CAD build for the part. Positions are in the model's coordinates, mm. A direction names the side the tool comes from. Round coordinates to 2 decimals unless told otherwise and drop trailing zeros. Loops run counter-clockwise (first coordinate to the right, second up) from the corner with the lowest first, then second, coordinate; pieces in that order, holes last. Notation, with made-up numbers: M -35.5,88.5 L -29.5,88.5 A26 cw -29.5,119.5 Z; hole C -28.5,32.5 d3. An arc over 180 degrees is marked long. One line per item, written item: value. Start each with the question number.
from build123d import *

# Parameters (mm, degrees)
EXTRUDE_1_DEPTH          = 8
CUT_EXTRUDE_1_DEPTH      = 24.556069282
CUT_EXTRUDE_2_REACH      = 25.556
SKETCH_3_W               = 11.85
SKETCH_3_H               = 2.762520892
SKETCH_3_H_2             = 2.75
CUT_EXTRUDE_3_DEPTH      = 10
CUT_EXTRUDE_3_DEPTH_BACK = 3
SKETCH_4_W               = 1.2
SKETCH_4_H               = 1.4
SKETCH_4_W_2             = 0.9
SKETCH_4_H_2             = 1.28
SKETCH_4_H_3             = 0.95
SKETCH_5_R               = 0.35
EXTRUDE_2_DEPTH          = 4.8
CUT_EXTRUDE_4_DEPTH      = 1
SKETCH_7_W               = 4.4
SKETCH_7_H               = 5.2
CUT_EXTRUDE_5_DEPTH      = 19.930728988
SKETCH_8_W               = 1.6
SKETCH_8_H               = 1.6
SKETCH_8_W_2             = 1.55
SKETCH_8_H_2             = 5.8
CUT_EXTRUDE_6_DEPTH      = 1.5


with BuildPart() as part:
    # 草图1 → 凸台-拉伸1 (new, symmetric)
    with BuildSketch(Plane.XY):
        Polygon((-0.75, 5.1), (0.8, 5.1), (0.8, 2.6), (0, 2.6), (0, -2.6), (3, -2.6), (3, -6.1), (0.15, -6.1), (0.15, -8.2), (-0.75, -8.2), (-0.75, -3.25), (-9.45, -3.25), (-9.45, -8.2), (-10.65, -8.2), (-10.65, -6.1), (-17.72, -6.1), (-17.72, -2.6), (-10.25, -2.6), (-10.25, 2.6), (-11.05, 2.6), (-11.05, 5.1), (-9.45, 5.1), (-9.45, 3.25), (-0.75, 3.25), align=None)
    extrude(amount=EXTRUDE_1_DEPTH, both=True)

    # 草图2 → 切除-拉伸1 (cut, through all)
    with BuildSketch(Plane(origin=(0, 5.1, 0), x_dir=(1, 0, 0), z_dir=(0, 1, 0))):
        Polygon((-11.05, 8.719427198), (-0.75, 8.719427198), (-0.75, 2.8), (-9.45, 2.8), (-9.45, 5.25), (-11.05, 5.25), align=None)
        Polygon((-11.05, -8), (-0.75, -8), (-0.75, -2.8), (-9.45, -2.8), (-9.45, -5.25), (-11.05, -5.25), align=None)
    extrude(amount=-CUT_EXTRUDE_1_DEPTH, mode=Mode.SUBTRACT)

    # 切除-拉伸2: up to this face of the body (flat: up to its plane)
    cut_extrude_2_end = Plane(part.part.faces().sort_by_distance((-14.112466991, -2.6, 0))[0])
    # 草图3 → 切除-拉伸2 (cut, up to the picked face)
    with BuildSketch(Plane(origin=(0, 5.1, 0), x_dir=(1, 0, 0), z_dir=(0, 1, 0)), mode=Mode.PRIVATE) as cut_extrude_2_sk1:
        with Locations((-5.125, 6.618739554)):
            Rectangle(SKETCH_3_W, SKETCH_3_H)
    cut_extrude_2_tool1 = split(extrude(cut_extrude_2_sk1.sketch, amount=-CUT_EXTRUDE_2_REACH, mode=Mode.PRIVATE), bisect_by=cut_extrude_2_end, keep=Keep.BOTH, mode=Mode.PRIVATE)
    # 草图3 → 切除-拉伸2 (cut, up to the picked face)
    with BuildSketch(Plane(origin=(0, 5.1, 0), x_dir=(1, 0, 0), z_dir=(0, 1, 0)), mode=Mode.PRIVATE) as cut_extrude_2_sk2:
        with Locations((-5.125, -6.625)):
            Rectangle(SKETCH_3_W, SKETCH_3_H_2)
    cut_extrude_2_tool2 = split(extrude(cut_extrude_2_sk2.sketch, amount=-CUT_EXTRUDE_2_REACH, mode=Mode.PRIVATE), bisect_by=cut_extrude_2_end, keep=Keep.BOTH, mode=Mode.PRIVATE)
    add(cut_extrude_2_tool1.solids().sort_by(Axis((-5.125, 5.1, -6.61874), (0, -1, 0)))[0], mode=Mode.SUBTRACT)
    add(cut_extrude_2_tool2.solids().sort_by(Axis((-5.125, 5.1, 6.625), (0, -1, 0)))[0], mode=Mode.SUBTRACT)

    # 草图4 → 切除-拉伸3 (cut, two sides: drawn at the far end of the back side and taken through both)
    with BuildSketch(Plane.XZ.offset(6.1).offset(-CUT_EXTRUDE_3_DEPTH_BACK)):
        with Locations((-10.05, 1.6)):
            Rectangle(SKETCH_4_W, SKETCH_4_H)
        with Locations((-10.05, -1.6)):
            Rectangle(SKETCH_4_W, SKETCH_4_H)
        with Locations((-0.3, 2.88)):
            Rectangle(SKETCH_4_W_2, SKETCH_4_H_2)
        with Locations((-0.3, -2.88)):
            Rectangle(SKETCH_4_W_2, SKETCH_4_H_2)
        with Locations((-0.3, 0)):
            Rectangle(SKETCH_4_W_2, SKETCH_4_H_2)
        with Locations((-0.3, 5.76)):
            Rectangle(SKETCH_4_W_2, SKETCH_4_H_2)
        with Locations((-0.3, -5.76)):
            Rectangle(SKETCH_4_W_2, SKETCH_4_H_2)
        with Locations((-10.05, 4.775)):
            Rectangle(SKETCH_4_W, SKETCH_4_H_3)
        with Locations((-10.05, -4.775)):
            Rectangle(SKETCH_4_W, SKETCH_4_H_3)
    extrude(amount=CUT_EXTRUDE_3_DEPTH + CUT_EXTRUDE_3_DEPTH_BACK, mode=Mode.SUBTRACT)

    # 草图5 → 凸台-拉伸2 (add)
    with BuildSketch(Plane.XZ.offset(6.1)):
        with Locations(Location((-15.65, 0, 0), (0, 0, 90))):
            Circle(SKETCH_5_R)
        with Locations(Location((-15.65, 3.2, 0), (0, 0, 90))):
            Circle(SKETCH_5_R)
        with Locations(Location((-15.65, 6.4, 0), (0, 0, 90))):
            Circle(SKETCH_5_R)
        with Locations(Location((-15.65, -3.2, 0), (0, 0, 90))):
            Circle(SKETCH_5_R)
        with Locations(Location((-15.65, -6.4, 0), (0, 0, 90))):
            Circle(SKETCH_5_R)
        with Locations(Location((1.75, 6.4, 0), (0, 0, 180))):
            Circle(SKETCH_5_R)
        with Locations(Location((1.75, 3.2, 0), (0, 0, 180))):
            Circle(SKETCH_5_R)
        with Locations(Location((1.75, 0, 0), (0, 0, 180))):
            Circle(SKETCH_5_R)
        with Locations(Location((1.75, -3.2, 0), (0, 0, 180))):
            Circle(SKETCH_5_R)
        with Locations(Location((1.75, -6.4, 0), (0, 0, 180))):
            Circle(SKETCH_5_R)
    extrude(amount=EXTRUDE_2_DEPTH)

    # 草图6 → 切除-拉伸4 (cut)
    with BuildSketch(Plane.XZ.offset(6.1)):
        Polygon((-16.22, 2.137501461), (-13.276335298, 2.137501461), (-15.965272543, 5.540797618), (-14.866770258, 6.408721998), (-11.492087758, 2.137501461), (-10.65, 2.137501461), (-10.65, 0.737501461), (-16.22, 0.737501461), align=None)
        Polygon((-16.22, -0.737501461), (-10.65, -0.737501461), (-10.65, -2.503069938), (-11.492087758, -2.503069938), (-14.964878351, -6.426327028), (-15.965272543, -5.540797618), (-13.276335298, -2.503069938), (-16.22, -2.503069938), align=None)
    extrude(amount=-CUT_EXTRUDE_4_DEPTH, mode=Mode.SUBTRACT)

    # 草图7 → 切除-拉伸5 (cut, through all)
    with BuildSketch(Plane.ZY.offset(10.25)):
        Rectangle(SKETCH_7_W, SKETCH_7_H)
    extrude(amount=-CUT_EXTRUDE_5_DEPTH, mode=Mode.SUBTRACT)

    # 草图8 → 切除-拉伸6 (cut)
    with BuildSketch(Plane(origin=(0, 5.1, 0), x_dir=(1, 0, 0), z_dir=(0, 1, 0))):
        with Locations((-10.25, 1.8)):
            Rectangle(SKETCH_8_W, SKETCH_8_H)
        with Locations((-10.25, -1.8)):
            Rectangle(SKETCH_8_W, SKETCH_8_H)
        with Locations((0.025, 0)):
            Rectangle(SKETCH_8_W_2, SKETCH_8_H_2)
    extrude(amount=-CUT_EXTRUDE_6_DEPTH, mode=Mode.SUBTRACT)


solid = part.part
(1) Mould opens along Y. For faces 5 (the flat face through (0, 5.1, 4)), 6 (the flat face through (-14.8, -5.6, 2.138)), 7 (the flat face through (-5, 2.6, 0)) say: pulls with the +Y half, pulls with the -Y half, needs draft (parallel to the pull), parting line crosses it, or undercut.
(2) Probe L1, parallel to X at y = 3.25, z = 3.5; L2, parallel to Z at x = -2, y = 1.75; L3, parallel to X at y = -6, z = 2. List the from-to ranges inside material, lowest first.
(3) Slice it at B-B, the plane y = 4.25. List the corners of the cut face in (x, z).
(4) Slice it at C-C, the plane y = -1.5. List the corners of the cut face in (x, z), and give its area (3 significant figures).
(5) Slice it at D-D, the plane x = 1.75. List the corners of the cut face in (y, z).
(6) Which spindle directions (+Z, -Z, +X, -X, +Y, -Y) get a long thin tool onto all of the face, cutting with end or side? Do faces 1 (the flat face through (0.8, 3, 0)), 2 (the flat face through (-10.25, 0, 4)), 3 (the flat face through (-10, -6, -0.9)), 4 (the flat face through (-10, -6, 4.3)). Say none if no direction does.
(7) Slice it at A-A, the plane z = 0. List the corners of the cut face in (x, y).
(8) Flat gauge pins, fed straight in: P1, Ø1.5, axis at x = -15, y = -1.5, coming from the -Z side; P2, Ø3.5, axis at y = 1, z = 3.5, coming from the +X side; P3, Ø0.8, axis at x = 0, y = 3, coming from the +Z side; P4, Ø6, axis at x = -5, z = 0.5, coming from the +Y side. Where does each tip first touch, or does it go through?
Check result:
1. face 5: pulls with the +Y half
1. face 6: needs draft
1. face 7: undercut
2. L1: x = -11.05 to -9.45, -0.75 to 0.8
2. L2: z = -2.8 to -2.2, 2.2 to 2.8
2. L3: x = -17.72 to -16.22, -0.75 to 3
3. outline: M -11.05,-5.24 L -9.45,-5.24 L -9.45,-2.6 L -11.05,-2.6 Z; M -11.05,-1 L -9.45,-1 L -9.45,1 L -11.05,1 Z; M -11.05,2.6 L -9.45,2.6 L -9.45,5.25 L -11.05,5.25 Z; M -0.75,-5.24 L 0.8,-5.24 L 0.8,-2.9 L -0.75,-2.9 Z; M -0.75,2.9 L 0.8,2.9 L 0.8,5.25 L -0.75,5.25 Z
4. outline: M -10.25,-5.24 L -9.45,-5.24 L -9.45,-2.8 L -0.75,-2.8 L -0.75,-5.24 L 0,-5.24 L 0,-2.2 L -10.25,-2.2 Z; M -10.25,2.2 L 0,2.2 L 0,5.25 L -0.75,5.25 L -0.75,2.8 L -9.45,2.8 L -9.45,5.25 L -10.25,5.25 Z
4. area: 19.9 mm^2
5. outline: M -10.9,-6.75 L -6.1,-6.75 L -6.1,-8 L -2.6,-8 L -2.6,8 L -6.1,8 L -6.1,6.75 L -10.9,6.75 L -10.9,6.05 L -6.1,6.05 L -6.1,3.55 L -10.9,3.55 L -10.9,2.85 L -6.1,2.85 L -6.1,0.35 L -10.9,0.35 L -10.9,-0.35 L -6.1,-0.35 L -6.1,-2.85 L -10.9,-2.85 L -10.9,-3.55 L -6.1,-3.55 L -6.1,-6.05 L -10.9,-6.05 Z
6. face 1: +Z, -Z, +X, +Y
6. face 2: +Z, -Z, -X
6. face 3: -Y
6. face 4: +Z, -Y
7. outline: M -17.72,-6.1 L -16,-6.1 L -16,-10.9 L -15.3,-10.9 L -15.3,-6.1 L -10.65,-6.1 L -10.65,-8.2 L -9.45,-8.2 L -9.45,-3.25 L -0.75,-3.25 L -0.75,-3.1 L 0.15,-3.1 L 0.15,-6.1 L 1.4,-6.1 L 1.4,-10.9 L 2.1,-10.9 L 2.1,-6.1 L 3,-6.1 L 3,-2.6 L -17.72,-2.6 Z; M -11.05,2.6 L 0.8,2.6 L 0.8,3.6 L -0.75,3.6 L -0.75,3.25 L -9.45,3.25 L -9.45,5.1 L -11.05,5.1 Z
8. P1: passes through
8. P2: stops at x = 0.8
8. P3: stops at z = 5.25
8. P4: stops at y = 3.25
